Geometry check sheet. Reference: drawing and pictorial views, mm from the part's lowest x, y, z. A direction names the side the tool comes from. Give positions to 0.01 mm unless a question says otherwise; leave off trailing zeros. Order: outer loops, then holes, each group sorted by start corner. A loop starts at its lowest first (then second) coordinate and runs counter-clockwise, first axis right, second up. Notation, with made-up numbers: (22.25, 1.25) - (58.25, 1.25) arc R6 cw to (58.25, 11.25) - close; hole circle Ø8 at (1, -21.75). An arc over 180 degrees is marked (long way). Answer in a Markdown table with one row per item.
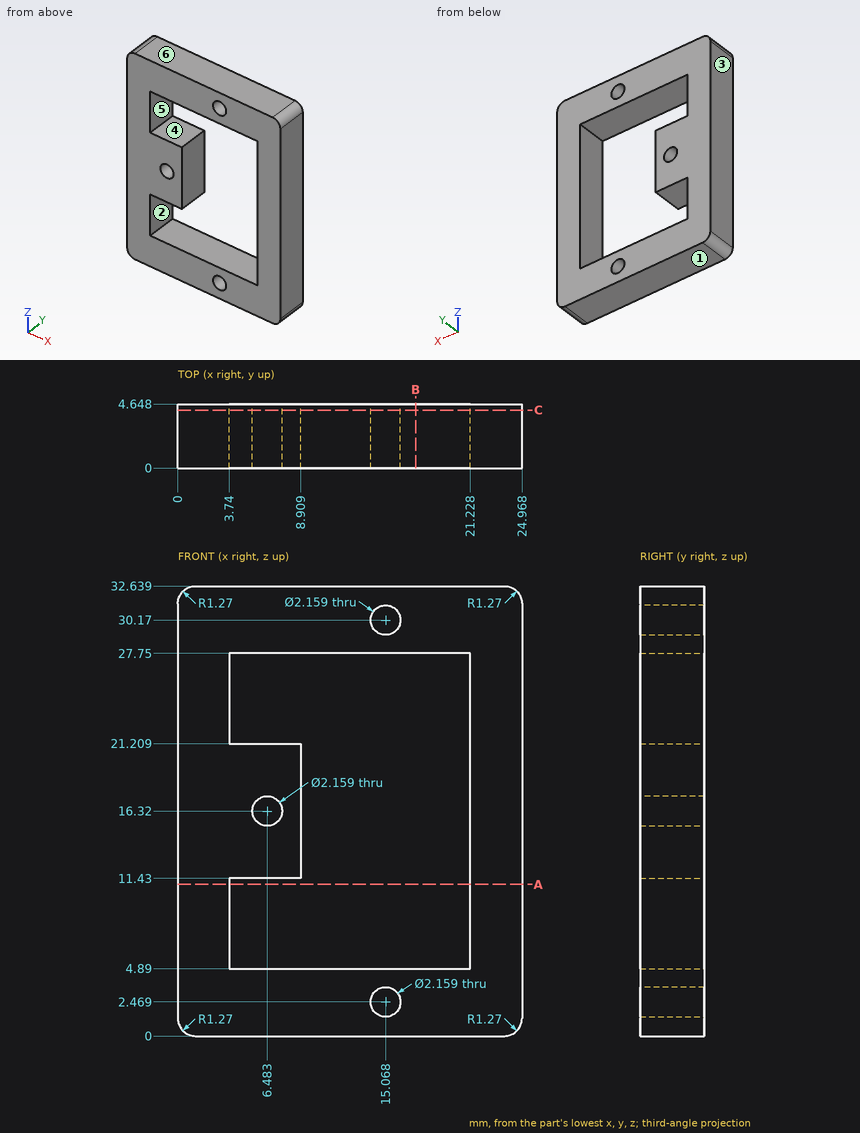
(1) Cross-section at C-C, the plane y = 4.2. Record the cut outline in (x, z).
Geometry says:
| item | result |
|---|---|
| outline | (0, 1.27) arc R1.27 ccw to (1.27, 0) - (23.7, 0) arc R1.27 ccw to (24.97, 1.27) - (24.97, 31.37) arc R1.27 ccw to (23.7, 32.64) - (1.27, 32.64) arc R1.27 ccw to (0, 31.37) - close; hole (3.74, 4.89) - (21.23, 4.89) - (21.23, 27.75) - (3.74, 27.75) - (3.74, 21.21) - (8.91, 21.21) - (8.91, 11.43) - (3.74, 11.43) - close; hole circle Ø2.16 at (6.48, 16.32); hole circle Ø2.16 at (15.07, 2.47); hole circle Ø2.16 at (15.07, 30.17) |
(2) Cross-section at B-B, the plane x = 17.25. Record the cut outline in (y, z).
Geometry says:
| item | result |
|---|---|
| outline | (0, 0) - (4.65, 0) - (4.65, 4.89) - (0, 4.89) - close; (0, 27.75) - (4.65, 27.75) - (4.65, 32.64) - (0, 32.64) - close |
(3) Mould release check, pull along X, two halves, no side actions. Record for the marked faces 1, 2, 3 and 4: pulls with the +X half, pulls with the -X half, needs draft (parallel to the pull), parting line crosses it, or undercut.
Geometry says:
| item | result |
|---|---|
| face 1 | needs draft |
| face 2 | undercut |
| face 3 | pulls with the -X half |
| face 4 | undercut |
(4) Access from +Z, -Z, +X, -X, +Y, -Y to the whole of each face (thin tool, end or side, straight path). Record for the marked faces 5 and 6.
Geometry says:
| item | result |
|---|---|
| face 5 | +Y, -Y |
| face 6 | +Z, +X, -X, +Y, -Y |
(5) Cross-section at A-A, the plane z = 11. Record the cut outline in (x, y).
Geometry says:
| item | result |
|---|---|
| outline | (0, 0) - (3.74, 0) - (3.74, 4.65) - (0, 4.65) - close; (21.23, 0) - (24.97, 0) - (24.97, 4.65) - (21.23, 4.65) - close |
(6) Gauge pin test, flat end, axial feed: P1, Ø3, axis at x = 15.07, z = 30.17, coming from the +Y side. Record the tip position at first contact, or that the pin passes through.
Geometry says:
| item | result |
|---|---|
| P1 | y = 4.65 |
(7) Thickness scan on L1, parallel to X at y = 1.65, z = 5; L2, parallel to Z at x = 20, y = 1.85; L3, parallel to X at y = 1.7, z = 20.5. Record the ranges inside material, lowest first.
Geometry says:
| item | result |
|---|---|
| L1 | 0 to 3.74, 21.23 to 24.97 |
| L2 | 0 to 4.89, 27.75 to 32.64 |
| L3 | 0 to 8.91, 21.23 to 24.97 |
